Input: part model. Units: mm. Frame: model coordinates. Face numbers are marked on the shaded views. A direction names the side the tool comes from. Give positions to 0.01 mm unless a question says otherwise; leave off trailing zeros. Order: outer loops, then holes, each group sorted by start corner. A loop starts at its lowest first (then second) coordinate and runs counter-clockwise, first axis right, second up. Notation, with made-up numbers: (-29.75, 59) - (14.25, 59) arc R9 ccw to (14.25, 76) - close; hole circle Ø2 at (-16, -18). An arc over 180 degrees is marked (long way). Answer in a Markdown table with one row per item. Add a question column.
1. Ray query, line 1 (X direction, y = -14.5, z = 45); line 2 (Z direction, x = 150, y = -102); line 3 (X direction, y = -96, z = 129.5). Return the intervals inside material, ascending. Write a range as [from, to].
2. Access query for the marked faces 4, 5, 6 and 7. Directions: +Z, -Z, +X, -X, +Y, -Y. A direction counts if a zero-diameter tool reaches every point of the face in a straight line with its end or side. Return the directions, or none.
3. Section query A-A on z = 19.5. Return loops of the section in (x, y).
4. Section query C-C on z = 120. Return loops of the section in (x, y).
5. Section query D-D on x = 31.5. Return loops of the section in (y, z).
6. Mould query, pull axis X, two halves, no side actions, for the marked faces 1, 2 and 3. Classes: released by +X, released by -X, zero draft, split by the parting line, or undercut.
7. Contact query for flat-ended pins moving along their axis: pin 1 (2 mm diameter, centred on y = -91, z = 68.5, fed in from +X); pin 2 (3 mm diameter, centred on x = 178.5, z = 138, fed in from -Y); pin 3 (1.9 mm diameter, centred on x = 181.5, y = 15.5, fed in from +Z); pin 4 (10 mm diameter, centred on y = -64, z = 22, fed in from -X). Output: stop coordinate, or through.
8. Section query B-B on y = 10. Return loops of the section in (x, z), and give its area (3 significant figures).
```python
from build123d import *

# Parameters (mm, degrees)
F1_DEPTH  = 10
F5_DEPTH  = 10
F4_W      = 1.2
F4_H      = 20
F12_DEPTH = 8
F13_W     = 22
F13_H     = 13.3
F14_DEPTH = 2
F17_DEPTH = 22
F19_ANGLE = -30
F21_DEPTH = 4


# Not quite as in the source:
# - the program builds the solid bodies; features that only make, move or delete a surface that nothing else refers to are left out


with BuildPart() as f1:
    # F0 (on Top) → F1 (new body)
    with BuildSketch(Plane.XY):
        Polygon((-21.2, 21.2), (21.2, 21.2), (21.2, -21.2), (-21.2, -21.2), (-21.2, -5), (-23.7, -5), (-23.7, -23.7), (23.7, -23.7), (23.7, 23.7), (-23.7, 23.7), (-23.7, 5), (-21.2, 5), align=None)
    extrude(amount=F1_DEPTH)



with BuildPart() as f5:
    # F4 (on line) → F5 (new body)
    with BuildSketch(Plane.YZ.offset(175)):
        with BuildLine():
            Line((15.5, 130), (15.5, 0))
            Line((15.5, 0), (31, 0))
            ThreePointArc((31, 0), (20.2857494387, 64.6079324383), (16.7, 130))
            Line((16.7, 130), (16.7, 150))
            Line((16.7, 150), (15.5, 150))
            Line((15.5, 150), (15.5, 130))
        make_face()
        with BuildLine():
            ThreePointArc((14.3, 130), (10.7142505613, 64.6079324383), (0, 0))
            Line((0, 0), (15.5, 0))
            Line((15.5, 0), (15.5, 130))
            Line((15.5, 130), (15.5, 150))
            Line((15.5, 150), (14.3, 150))
            Line((14.3, 150), (14.3, 130))
        make_face()
    extrude(amount=F5_DEPTH)

    # F4 (on line) → F5, piece 2 (join)
    with BuildSketch(Plane.YZ.offset(175)):
        with BuildLine():
            Line((-15.5, 0), (0, 0))
            ThreePointArc((0, 0), (-10.7142505613, 64.6079324383), (-14.3, 130))
            Line((-14.3, 130), (-15.5, 130))
            Line((-15.5, 130), (-15.5, 0))
        make_face()
        with BuildLine():
            Line((-31, 0), (-15.5, 0))
            Line((-15.5, 0), (-15.5, 130))
            Line((-15.5, 130), (-16.7, 130))
            ThreePointArc((-16.7, 130), (-20.2857494387, 64.6079324383), (-31, 0))
        make_face()
        with Locations((-14.9, 140)):
            Rectangle(F4_W, F4_H)
        with Locations((-16.1, 140)):
            Rectangle(F4_W, F4_H)
    extrude(amount=F5_DEPTH)


with BuildPart() as f12:
    # F11 (on line) → F12 (new body)
    with BuildSketch(Plane.XY.offset(150)):
        Polygon((141.5544456623, -82.85), (161.5544456623, -82.85), (161.5544456623, -84.8), (163.5544456623, -84.8), (163.5544456623, -80.85), (141.5544456623, -80.85), align=None)
    extrude(amount=F12_DEPTH)



with BuildPart() as f12b:
    # F11 (on line) → F12, piece 2 (new body)
    with BuildSketch(Plane.XY.offset(150)):
        Polygon((161.5544456623, -92.15), (141.5544456623, -92.15), (141.5544456623, -94.15), (163.5544456623, -94.15), (163.5544456623, -90.2), (161.5544456623, -90.2), align=None)
    extrude(amount=F12_DEPTH)


with BuildPart() as f12_1:
    add(f12.part)

    add(f12b.part)  # F14 merges F12b
    # F13 (on line) → F14 (join)
    with BuildSketch(Plane.XY.offset(150)):
        with Locations((152.5544456623, -87.5)):
            Rectangle(F13_W, F13_H)
    extrude(amount=-F14_DEPTH)

    # F16 (on face) → F17 (join)
    with BuildSketch(Plane(origin=(163.5544456623, 0, 0), x_dir=(0, -1, 0), z_dir=(-1, 0, 0))):
        with BuildLine():
            Line((87.5, 0), (87.5, 148))
            Line((87.5, 148), (80.85, 148))
            ThreePointArc((80.85, 148), (79.1866617309, 73.9253374966), (74.2, 0))
            Line((74.2, 0), (87.5, 0))
        make_face()
        with BuildLine():
            Line((94.15, 148), (87.5, 148))
            Line((87.5, 148), (87.5, 0))
            Line((87.5, 0), (100.8, 0))
            ThreePointArc((100.8, 0), (95.8133382691, 73.9253374966), (94.15, 148))
        make_face()
    extrude(amount=F17_DEPTH)

    # F18: union 


with BuildPart() as f12_2:
    # F19: moved
    add(f12_1.part.rotate(Axis((151.5544456623, -87.5, 75), (0, 0, 1)), F19_ANGLE))


with BuildPart() as f1_1:
    add(f1.part)

    add(f5.part)  # F21 merges F5

    add(f12_2.part)  # F21 merges F12
    # F20 (on Top) → F21 (join)
    with BuildSketch(Plane.XY):
        Polygon((-25.7, 25.7), (-25.7, -25.7), (25.7, -25.7), (25.7, -17.1473029949), (140.1621408169, -83.2320508076), (133.5121408169, -94.7501886779), (156.0288013153, -107.7501886779), (170.4353579421, -82.7973006382), (187, -31.313824878), (187, 0), (187, 33), (173, 33), (173, 2), (25.7, 2), (25.7, 25.7), align=None)
        Polygon((23.7, 0), (175, 0), (175, 31), (185, 31), (185, 0), (185, -31), (168.5967505077, -81.9818621297), (155.2967505077, -105.0181378703), (136.2441916244, -94.0181378703), (142.8941916244, -82.5), (23.7, -13.6832013798), (23.7, -23.7), (-23.7, -23.7), (-23.7, 23.7), (23.7, 23.7), align=None, mode=Mode.SUBTRACT)
        Polygon((175, 31), (175, 0), (23.7, 0), (23.7, 23.7), (-23.7, 23.7), (-23.7, -23.7), (23.7, -23.7), (23.7, -13.6832013798), (142.8941916244, -82.5), (136.2441916244, -94.0181378703), (155.2967505077, -105.0181378703), (168.5967505077, -81.9818621297), (185, -31), (185, 0), (185, 31), align=None)
    extrude(amount=-F21_DEPTH)


solid = f1_1.part
```
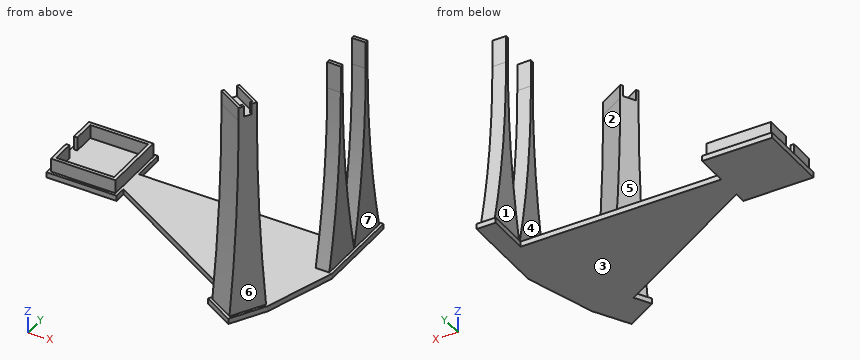
Answer:
| question | item | result |
|---|---|---|
| 1 | line 1 | x = [175, 185] |
| 1 | line 2 | z = [-4, 0] |
| 1 | line 3 | x = [152.77, 160.5] |
| 2 | face 4 | +Z, +Y, -Y |
| 2 | face 5 | +Z, -X, +Y |
| 2 | face 6 | +Z, +X, -Y |
| 2 | face 7 | +Z, +X, +Y, -Y |
| 3 | outline | (137.06, -92.6) - (156.12, -103.6) - (167.78, -83.4) - (148.72, -72.4) - close; (175, -27) - (185, -27) - (185, -4) - (175, -4) - close; (175, 4) - (185, 4) - (185, 27) - (175, 27) - close |
| 4 | outline | (139.45, -88.46) - (158.5, -99.46) - (165.39, -87.54) - (146.34, -76.54) - close; (175, -16.78) - (185, -16.78) - (185, -14.22) - (175, -14.22) - close; (175, 14.22) - (185, 14.22) - (185, 16.78) - (175, 16.78) - close |
| 5 | outline | (-20.5, -4) - (2, -4) - (2, 0) - (-20.5, 0) - close |
| 6 | face 1 | undercut |
| 6 | face 2 | released by +X |
| 6 | face 3 | zero draft |
| 7 | pin 1 | stops at x = 163.97 |
| 7 | pin 2 | stops at y = -16.7 |
| 7 | pin 3 | stops at z = 150 |
| 7 | pin 4 | passes through |
| 8 | outline | (-25.7, -4) - (25.7, -4) - (25.7, 0) - (23.7, 0) - (23.7, 10) - (21.2, 10) - (21.2, 0) - (-21.2, 0) - (-21.2, 10) - (-23.7, 10) - (-23.7, 0) - (-25.7, 0) - close; (173, -4) - (187, -4) - (187, 0) - (185, 0) - (185, 58.41) - (175, 58.41) - (175, 0) - (173, 0) - close |
| 8 | area | 896 mm² |
